Design review of the part built by this model. Coordinates are the model's own, in mm. A direction names the side the tool comes from. Give positions to 0.01 mm unless a question says otherwise; leave off trailing zeros. Order: outer loops, then holes, each group sorted by start corner. A loop starts at its lowest first (then second) coordinate and runs counter-clockwise, first axis right, second up. Notation, with made-up numbers: (-32, 75.5) -> (-11, 75.5) arc R14 ccw to (-11, 97.5) -> close; hole circle Ø4 at (62, -28.75). An arc over 180 degrees is marked (long way). One line per item, written item: value. Start each with the question number.
1) Wall thickness on line 1 along X through (y, z) = (3.5, 65.5); line 2 along X through (y, z) = (5, 74.5); line 3 along Z through (x, y) = (-21.5, 1.5): over which ranges is each line inside the solid? List them lowest first. Write a range as from..to.
2) For pin 1 (1 mm diameter, centred on x = -24.5, y = 2, fed in from -Z); pin 2 (4 mm diameter, centred on x = -18, y = 5, fed in from -Z); pin 3 (3 mm diameter, centred on x = -19.5, y = 2, fed in from -Z), all flat-tipped, find the tip position at first contact; note any pin that passes through.
3) Tool access review of faces 1 (the face through (-23.78, 7.64, 84.25)), 2 (the face through (-16.679, 0.247, 72.992)), 3 (the face through (-25.64, 0.25, 72.14)), 4 (the face through (-19.405, 3.951, 72.657)): name each direction out of +Z, -Z, +X, -X, +Y, -Y from which nothing blocks a thin tool from reaching the whole face with its end or side.
4) Consider section A-A (y = 3). State the section outline as (x, z) points.
5) Consider section B-B (z = 69). State the section outline as (x, y) points, plus the area to 3 significant figures.
6) The part is to be moulded in two halves that separate along Z. For faces 5 (the face through (-16.427, 3.951, 73.023)), 6 (the face through (-18, 0, 72)), 7 (the face through (-21.01, 0.36, 60.58)), say which applies: released by +Z, released by -Z, zero draft, split by the parting line, or undercut.
from build123d import *

# Parameters (mm, degrees)
BOSS_EXTRUDE1_DEPTH = 8
CHAMFER1_SIZE       = 0.5


with BuildPart() as part:
    # Sketch1 → Boss-Extrude1 (new body)
    with BuildSketch(Plane(origin=(0, 0, 0), x_dir=(1, 0, 0), z_dir=(0, 1, 0))):
        with BuildLine():
            Line((-29.422447973, -80.393109081), (-27.283313621, -62.971257862))
            ThreePointArc((-27.283313621, -62.971257862), (-20.596820651, -57.747197013), (-15.372759802, -64.433689983))
            Line((-15.372759802, -64.433689983), (-17.511894154, -81.855541202))
            ThreePointArc((-17.511894154, -81.855541202), (-24.198387124, -87.079602051), (-29.422447973, -80.393109081))
        make_face()
        with BuildLine():
            Line((-26.444809519, -80.758717111), (-24.305675167, -63.336865893))
            ThreePointArc((-24.305675167, -63.336865893), (-20.962428681, -60.724835468), (-18.350398257, -64.068081953))
            Line((-18.350398257, -64.068081953), (-20.489532609, -81.489933172))
            ThreePointArc((-20.489532609, -81.489933172), (-23.832779094, -84.101963596), (-26.444809519, -80.758717111))
        make_face(mode=Mode.SUBTRACT)
    extrude(amount=BOSS_EXTRUDE1_DEPTH)

    # Chamfer1
    chamfer1_edges = [part.edges().sort_by_distance(p)[0] for p in [
        (-20.596820651, 8, 57.747197013),
        (-28.352880797, 8, 71.682183472),
        (-20.962428681, 0, 60.724835468),
        (-25.375242343, 0, 72.047791502),
        (-23.832779094, 0, 84.101963596),
        (-19.419965433, 0, 72.779007562),
        (-20.962428681, 8, 60.724835468),
        (-25.375242343, 8, 72.047791502),
        (-23.832779094, 8, 84.101963596),
        (-19.419965433, 8, 72.779007562),
        (-24.198387124, 8, 87.079602051),
        (-28.352880797, 0, 71.682183472),
        (-20.596820651, 0, 57.747197013),
        (-16.442326978, 0, 73.144615593),
        (-24.198387124, 0, 87.079602051),
        (-16.442326978, 8, 73.144615593),
    ]]
    chamfer(chamfer1_edges, length=CHAMFER1_SIZE)


solid = part.part
Checked values:
1. line 1: x = -27.59..-24.57, -18.53..-15.5
1. line 2: x = -28.7..-25.68, -19.63..-16.61
1. line 3: z = 57.7..60.71, 83.39..86.79
2. pin 1: stops at z = 58.33
2. pin 2: stops at z = 57.85
2. pin 3: stops at z = 57.71
3. face 1: +Y
3. face 2: +Z, +X, -Y
3. face 3: -Y
3. face 4: +Y, -Y
4. outline: (-29.42, 80.39) -> (-27.28, 62.97) arc R6 ccw to (-15.37, 64.43) -> (-17.51, 81.86) arc R6 ccw to start; hole (-26.44, 80.76) -> (-24.31, 63.34) arc R3 ccw to (-18.35, 64.07) -> (-20.49, 81.49) arc R3 ccw to start
5. outline: (-28.02, 0.5) -> (-27.52, 0) -> (-25.5, 0) -> (-25, 0.5) -> (-25, 7.5) -> (-25.5, 8) -> (-27.52, 8) -> (-28.02, 7.5) -> close; (-18.96, 0.5) -> (-18.45, 0) -> (-16.44, 0) -> (-15.93, 0.5) -> (-15.93, 7.5) -> (-16.44, 8) -> (-18.45, 8) -> (-18.96, 7.5) -> close
5. area: 47.4 mm^2
6. face 5: released by +Z
6. face 6: zero draft
6. face 7: undercut
